Build history of the part. All positions in model axes, mm. A direction names the side the tool comes from. Give positions to 0.01 mm unless a question says otherwise; leave off trailing zeros. Loops run counter-clockwise (first coordinate to the right, second up) from the corner with the lowest first, then second, coordinate; pieces in that order, holes last. Notation, with made-up numbers: M 5,29.25 L 35,29.25 A18 ccw 35,47.25 Z; hole C -24.75,78 d8. An arc over 180 degrees is marked long. Put each result on its own line as item: value.
```python
from build123d import *

# Parameters (mm, degrees)
F1_DEPTH     = 2
F2_R         = 1
F4_DEPTH     = 2.25
F6_DEPTH     = 2.2
F7_R         = 2
F8_DEPTH     = 25
F9_R         = 3.25
F9_R_2       = 2
F10_DEPTH    = 2.25
F12_DEPTH    = 4.65
F14_DEPTH    = 3.5
F16_DEPTH    = 1
F17_R        = 1.75
F18_DEPTH    = 25
F20_DEPTH    = 3.15
F21_W        = 9.561190108
F21_H        = 6.25
F22_DEPTH    = 4.45
F23_T4_DEPTH = 21.0051794045
F23_T9_DEPTH = 21.0051794045
F24_SIZE     = 1
F26_DEPTH    = 4.25
F27_R        = 1


# Not quite as in the source:
# - a fillet or chamfer that OpenCascade refuses, or shapes differently, is made with other operations: its cross-section is extruded or revolved along the edge and cut away or added
# - a pattern or mirror of a feature is missing from the dataset's text; its kind, count and spacing are read off the source's solid


with BuildPart() as f1:
    # F0 (on Top) → F1 (new body)
    with BuildSketch(Plane.XY):
        with BuildLine():
            Line((21.9083046755, 12.75), (-21.9083046755, 12.75))
            ThreePointArc((-21.9083046755, 12.75), (-23, 0), (-21.9083046755, -12.75))
            Line((-21.9083046755, -12.75), (21.9083046755, -12.75))
            ThreePointArc((21.9083046755, -12.75), (23, 0), (21.9083046755, 12.75))
        make_face()
    extrude(amount=F1_DEPTH)

    # F2
    f2_edges = [f1.edges().sort_by_distance(p)[0] for p in [
        (-21.908305, 12.75, 1),
        (21.908305, 12.75, 1),
        (-21.908305, -12.75, 1),
        (21.908305, -12.75, 1),
    ]]
    fillet(f2_edges, radius=F2_R)

    # F3 (on face) → F4 (join)
    with BuildSketch(Plane(origin=(0, 0, 0), x_dir=(1, 0, 0), z_dir=(0, 0, -1))):
        with BuildLine():
            Line((11.5, 12.75), (-21.061190108, 12.75))
            ThreePointArc((-21.061190108, 12.75), (-21.7097331737, 12.5111779634), (-22.0485034879, 11.9087837838))
            ThreePointArc((-22.0485034879, 11.9087837838), (-23, 0), (-22.0485034879, -11.9087837838))
            ThreePointArc((-22.0485034879, -11.9087837838), (-21.7097331737, -12.5111779634), (-21.061190108, -12.75))
            Line((-21.061190108, -12.75), (11.5, -12.75))
            Line((11.5, -12.75), (11.5, 12.75))
        make_face()
    extrude(amount=F4_DEPTH)

    # F5 (on face) → F6 (join)
    with BuildSketch(Plane(origin=(0, 0, -2.25), x_dir=(1, 0, 0), z_dir=(0, 0, -1))):
        with BuildLine():
            ThreePointArc((-22.0485034879, -11.9087837838), (-21.7097331737, -12.5111779634), (-21.061190108, -12.75))
            Line((-21.061190108, -12.75), (-12.5, -12.75))
            Line((-12.5, -12.75), (-12.5, 12.75))
            Line((-12.5, 12.75), (-21.061190108, 12.75))
            ThreePointArc((-21.061190108, 12.75), (-21.7097331737, 12.5111779634), (-22.0485034879, 11.9087837838))
            ThreePointArc((-22.0485034879, 11.9087837838), (-23, 0), (-22.0485034879, -11.9087837838))
        make_face()
    extrude(amount=F6_DEPTH)

    # F7 (on face) → F8 (cut)
    with BuildSketch(Plane(origin=(0, 0, -2.25), x_dir=(1, 0, 0), z_dir=(0, 0, -1))):
        with Locations((-7.5, 0)):
            Circle(F7_R)
    extrude(amount=-F8_DEPTH, mode=Mode.SUBTRACT)

    # F9 (on face) → F10 (cut)
    with BuildSketch(Plane.XY.offset(2)):
        with Locations((-7.5, 0)):
            Circle(F9_R)
        with Locations((-7.5, 0)):
            Circle(F9_R_2, mode=Mode.SUBTRACT)
    extrude(amount=-F10_DEPTH, mode=Mode.SUBTRACT)

    # F11 (on face) → F12 (cut)
    with BuildSketch(Plane.XY.offset(2)):
        Polygon((-17.9767161827, 6.3967091968), (-22.7267161827, 6.3967091968), (-22.7267161827, -6.3967091968), (-18.3871376794, -6.3967091968), align=None)
        with BuildLine():
            ThreePointArc((-22.7267161827, -6.3967091968), (-23, 0), (-22.7267161827, 6.3967091968))
            Line((-22.7267161827, 6.3967091968), (-24.9030976, 6.3967091968))
            Line((-24.9030976, 6.3967091968), (-24.9030976, -6.3967091968))
            Line((-24.9030976, -6.3967091968), (-23.1371376794, -6.3967091968))
            Line((-23.1371376794, -6.3967091968), (-22.7267161827, -6.3967091968))
        make_face()
        Polygon((-22.7267161827, -6.3967091968), (-22.7267161827, 6.3967091968), (-24.9030976, 6.3967091968), (-24.9030976, -6.3967091968), (-23.1371376794, -6.3967091968), align=None)
    extrude(amount=-F12_DEPTH, mode=Mode.SUBTRACT)

    # F13 (on face) → F14 (cut)
    with BuildSketch(Plane.XY.offset(2)):
        with BuildLine():
            Line((-8.0183982933, 4.9370567441), (-18.0132564134, 5.2576985384))
            Line((-18.0132564134, 5.2576985384), (-18.3403110436, -4.9370567441))
            Line((-18.3403110436, -4.9370567441), (-8.3454529235, -5.2576985384))
            Line((-8.3454529235, -5.2576985384), (-8.2780130541, -3.1555024462))
            ThreePointArc((-8.2780130541, -3.1555024462), (-10.748328889, 0.1042085831), (-8.074160142, 3.1988810749))
            Line((-8.074160142, 3.1988810749), (-8.0183982933, 4.9370567441))
        make_face()
    extrude(amount=-F14_DEPTH, mode=Mode.SUBTRACT)

    # F15 (on face) → F16 (cut)
    with BuildSketch(Plane.XY.offset(2)):
        with BuildLine():
            ThreePointArc((7.2010516835, -2.053352114), (7.5517942695, -2.0743534785), (7.9010516835, -2.0358739026))
            ThreePointArc((7.9010516835, -2.0358739026), (9.575, 0), (7.9010516835, 2.0358739026))
            ThreePointArc((7.9010516835, 2.0358739026), (7.5517942695, 2.0743534785), (7.2010516835, 2.053352114))
            ThreePointArc((7.2010516835, 2.053352114), (6.646380727, 1.8912850491), (6.1579127796, 1.5825381173))
            Line((6.1579127796, 1.5825381173), (6.1579127796, 4.5080841794))
            Line((6.1579127796, 4.5080841794), (-8.312298453, 4.5080841794))
            Line((-8.312298453, 4.5080841794), (-8.312298453, -4.22422681))
            Line((-8.312298453, -4.22422681), (3.735084728, -4.22422681))
            Line((3.735084728, -4.22422681), (3.735084728, -6.8032004514))
            ThreePointArc((3.735084728, -6.8032004514), (4.0668227554, -10.9249796186), (4.435084728, -6.8063030421))
            Line((4.435084728, -6.8063030421), (4.435084728, -4.22422681))
            Line((4.435084728, -4.22422681), (6.1579127796, -4.22422681))
            Line((6.1579127796, -4.22422681), (6.1579127796, -1.5825381173))
            ThreePointArc((6.1579127796, -1.5825381173), (6.646380727, -1.8912850491), (7.2010516835, -2.053352114))
        make_face()
    extrude(amount=-F16_DEPTH, mode=Mode.SUBTRACT)

    # F17 (on face) → F18 (cut)
    with BuildSketch(Plane.XY.offset(2)):
        with Locations((-4.5, 7)):
            Circle(F17_R)
        with Locations((-4.5, -7)):
            Circle(F17_R)
    extrude(amount=-F18_DEPTH, mode=Mode.SUBTRACT)

    # F19 (on face) → F20 (cut)
    with BuildSketch(Plane(origin=(0, 0, -2.25), x_dir=(1, 0, 0), z_dir=(0, 0, -1))):
        Polygon((-2.4359727876, 10.575), (-6.5640272124, 10.575), (-8.6280544247, 7), (-6.5640272124, 3.425), (-2.4359727876, 3.425), (-0.3719455753, 7), align=None)
        Polygon((-2.4359727876, -3.425), (-6.5640272124, -3.425), (-8.6280544247, -7), (-6.5640272124, -10.575), (-2.4359727876, -10.575), (-0.3719455753, -7), align=None)
    extrude(amount=-F20_DEPTH, mode=Mode.SUBTRACT)

    # F21 (on face) → F22 (join, through all)
    with BuildSketch(Plane(origin=(0, 0, 0), x_dir=(1, 0, 0), z_dir=(0, 0, -1))):
        with Locations((16.280595054, 9.625)):
            Rectangle(F21_W, F21_H)
        with Locations((16.280595054, -9.625)):
            Rectangle(F21_W, F21_H)
    extrude(amount=F22_DEPTH)

    # F23: chamfer of 4.45 on 2 edges, made by hand


with BuildPart() as f23_tool2:
    # F23_s3 → F23_t4 (new body)
    with BuildSketch(Plane.YZ.offset(11.5)):
        Polygon((-6.5, 0), (-10.95, -4.45), (-6.5, -4.45), align=None)
    extrude(amount=F23_T4_DEPTH)

    split(bisect_by=Plane.XY, keep=Keep.BOTTOM)


with BuildPart() as f1_1:
    add(f1.part)

    # F23_t1: cut F23_tool2
    add(f23_tool2.part, mode=Mode.SUBTRACT)


with BuildPart() as f23_tool7:
    # F23_s8 → F23_t9 (new body)
    with BuildSketch(Plane.YZ.offset(32.5051794045)):
        Polygon((10.95, -4.45), (6.5, 0), (6.5, -4.45), align=None)
    extrude(amount=-F23_T9_DEPTH)

    split(bisect_by=Plane.XY, keep=Keep.BOTTOM)


with BuildPart() as f1_2:
    add(f1_1.part)

    # F23_t6: cut F23_tool7
    add(f23_tool7.part, mode=Mode.SUBTRACT)

    # F24
    f24_edges = [f1_2.edges().sort_by_distance(p)[0] for p in [
        (-16.780595, -12.75, -4.45),
        (-16.780595, 12.75, -4.45),
        (-21.709733, -12.511178, -4.45),
        (-23, 0, -4.45),
        (-21.709733, 12.511178, -4.45),
    ]]
    chamfer(f24_edges, length=F24_SIZE)

    # F25 (on face) → F26 (join, through all)
    with BuildSketch(Plane.XY.offset(2)):
        with BuildLine():
            Line((-21.061190108, 17.75), (-21.061190108, 12.75))
            Line((-21.061190108, 12.75), (-4.561190108, 12.75))
            ThreePointArc((-4.561190108, 12.75), (-12.2301209331, 14.0351006072), (-19.061190108, 17.75))
            Line((-19.061190108, 17.75), (-21.061190108, 17.75))
        make_face()
    f26 = extrude(amount=-F26_DEPTH)

    # F26_copies: F26 across plane
    add(f26.mirror(Plane(origin=(0, 0, 0), x_dir=(0, 0, -1), z_dir=(0, -1, 0))))

    # F27
    f27_edges = [f1_2.edges().sort_by_distance(p)[0] for p in [
        (-19.06119, 17.75, -0.125),
        (-19.06119, -17.75, -0.125),
    ]]
    fillet(f27_edges, radius=F27_R)


solid = f1_2.part
```
Q1. Slice it at A-A (x = 14). List the corners of the cut face in (y, z).
Here are the results:
outline: M -12.75,-4.45 L -10.95,-4.45 L -6.5,0 L 6.5,0 L 10.95,-4.45 L 12.75,-4.45 L 12.75,2 L -12.75,2 Z
Q2. Slice it at C-C (x = 5). List the corners of the cut face in (y, z).
Here are the results:
outline: M -12.75,-2.25 L 12.75,-2.25 L 12.75,2 L 4.51,2 L 4.51,1 L -4.22,1 L -4.22,2 L -6.99,2 L -6.99,1 L -10.71,1 L -10.71,2 L -12.75,2 Z
Q3. Probe line 1 (Y direction, x = -4.5, z = 1.35); line 2 (Y direction, x = 18, z = -2.25); line 3 (Y direction, x = -21, z = -2). List the from-to ranges inside material, lowest first. Write a range as from..to.
Here are the results:
line 1: -12.75..-8.75, -5.25..-4.22, 4.51..5.25, 8.75..12.75
line 2: -12.75..-8.75, 8.75..12.75
line 3: -17.75..-6.4, 6.4..17.75
Q4. Slice it at D-D (y = -13.5). List the corners of the cut face in (x, z).
Here are the results:
outline: M -21.06,-2.25 L -10.45,-2.25 L -10.45,2 L -21.06,2 Z
Q5. Slice it at B-B (y = 0). List the corners of the cut face in (x, z) (3 decimals).
Here are the results:
outline: M -23,-3.45 L -22,-4.45 L -12.5,-4.45 L -12.5,-2.25 L -9.5,-2.25 L -9.5,-0.25 L -10.75,-0.25 L -10.75,-1.5 L -18.182,-1.5 L -18.182,-2.65 L -23,-2.65 Z; M -5.5,-2.25 L 11.5,-2.25 L 11.5,0 L 23,0 L 23,2 L 9.575,2 L 9.575,1 L -4.25,1 L -4.25,-0.25 L -5.5,-0.25 Z
Q6. Tool access for faces 4 (the flat face through (11.5, 0, -1)), 5 (the flat face through (21.061, -10, -2)), 6 (the flat face through (-4, -10.575, -1)): list every direction of +Z, -Z, +X, -X, +Y, -Y with a clear straight run to the whole face (end or side of a thin tool).
Here are the results:
face 4: -Z, +X
face 5: -Z, +X, +Y, -Y
face 6: -Z
Q7. Mould opens along Y. For faces 1 (the cylindrical face through (3.981, -10.923, 1.507)), 2 (the cylindrical face through (23, 0, 1)), 3 (the flat face through (-16.7, -12.3, -3.9)) say: pulls with the +Y half, pulls with the -Y half, needs draft (parallel to the pull), parting line crosses it, or undercut.
Here are the results:
face 1: undercut
face 2: parting line crosses it
face 3: pulls with the -Y half
Q8. Drop flat-ended pins along their axis: pin 1 Ø1.1 at (y, z) = (1.5, -1.5) entering from +X; pin 2 Ø4 at (x, y) = (-4.5, 7) entering from -Z; pin 3 Ø0.8 at (y, z) = (-5, 1.5) entering from -X. Give the stop position or say it passes through.
Here are the results:
pin 1: x = 11.5
pin 2: z = 0.9
pin 3: x = -18.36
